```python
from build123d import *

# Parameters (mm, degrees)
SKETCH3_W                       = 80
SKETCH3_H                       = 80
SKETCH3_W_2                     = 60
SKETCH3_H_2                     = 60
BOSS_EXTRUDE2_DEPTH             = 1600
SKETCH7_W                       = 60
SKETCH7_H                       = 60
BOSS_EXTRUDE3_DEPTH             = 5
BOSS_EXTRUDE4_REACH             = 1610.361
SKETCH8_W                       = 105
SKETCH8_H                       = 5
BOSS_EXTRUDE4_DIRECTION_2_REACH = 1610.361
CUT_EXTRUDE1_DEPTH              = 5
CUT_EXTRUDE2_REACH              = 1612.59
FILLET1_R                       = 5
FILLET1_OF_MIRROR1_R            = 5
FILLET1_OF_MIRROR2_R            = 5


with BuildPart() as part:
    # Sketch3 → Boss-Extrude2 (new body)
    with BuildSketch(Plane(origin=(0, 0, 0), x_dir=(0, 0, -1), z_dir=(1, 0, 0))):
        with Locations((40, 40)):
            Rectangle(SKETCH3_W, SKETCH3_H)
        with Locations((40, 40)):
            Rectangle(SKETCH3_W_2, SKETCH3_H_2, mode=Mode.SUBTRACT)
    extrude(amount=BOSS_EXTRUDE2_DEPTH)

    # Sketch7 → Boss-Extrude3 (add)
    with BuildSketch(Plane(origin=(1495, 0, 0), x_dir=(0, 0, -1), z_dir=(1, 0, 0))):
        Polygon((-60, 85), (140, 85), (140, 5), (90, -35), (-10, -35), (-60, 5), align=None)
        with Locations((40, 40)):
            Rectangle(SKETCH7_W, SKETCH7_H, mode=Mode.SUBTRACT)
    boss_extrude3 = extrude(amount=BOSS_EXTRUDE3_DEPTH)

    # Boss-Extrude4: up to this face of the body (flat: up to its plane)
    boss_extrude4_end = Plane(part.part.faces().sort_by_distance((1497.5, 45, -140))[0])
    # Sketch8 → Boss-Extrude4 (add, up to the picked face)
    with BuildSketch(Plane(origin=(0, 0, -80), x_dir=(-1, 0, 0), z_dir=(0, 0, -1)), mode=Mode.PRIVATE) as boss_extrude4_sk1:
        with Locations((-1447.5, 82.5)):
            Rectangle(SKETCH8_W, SKETCH8_H)
    boss_extrude4_tool1 = split(extrude(boss_extrude4_sk1.sketch, amount=BOSS_EXTRUDE4_REACH, mode=Mode.PRIVATE), bisect_by=boss_extrude4_end, keep=Keep.BOTH, mode=Mode.PRIVATE)
    boss_extrude4 = boss_extrude4_tool1.solids().sort_by(Axis((1447.5, 82.5, -80), (0, 0, -1)))[0]
    add(boss_extrude4)

    # Boss-Extrude4 direction 2: up to this face of the body (flat: up to its plane)
    boss_extrude4_direction_2_end = Plane(part.part.faces().sort_by_distance((1497.5, 45, 60))[0])
    # Sketch8 → Boss-Extrude4 direction 2 (add, up to the picked face)
    with BuildSketch(Plane(origin=(0, 0, -80), x_dir=(-1, 0, 0), z_dir=(0, 0, -1)), mode=Mode.PRIVATE) as boss_extrude4_direction_2_sk1:
        with Locations((-1447.5, 82.5)):
            Rectangle(SKETCH8_W, SKETCH8_H)
    boss_extrude4_direction_2_tool1 = split(extrude(boss_extrude4_direction_2_sk1.sketch, amount=-BOSS_EXTRUDE4_DIRECTION_2_REACH, mode=Mode.PRIVATE), bisect_by=boss_extrude4_direction_2_end, keep=Keep.BOTH, mode=Mode.PRIVATE)
    boss_extrude4_direction_2 = boss_extrude4_direction_2_tool1.solids().sort_by(Axis((1447.5, 82.5, -80), (0, 0, 1)))[0]
    add(boss_extrude4_direction_2)

    # Sketch9 → Cut-Extrude1 (cut)
    with BuildSketch(Plane(origin=(0, 85, 0), x_dir=(1, 0, 0), z_dir=(0, 1, 0))):
        with BuildLine():
            Line((1395, 80), (1400.801257358, 71.298113962))
            ThreePointArc((1400.801257358, 71.298113962), (1403.927300662, 64.675212774), (1405, 57.430609057))
            Line((1405, 57.430609057), (1405, 22.569390943))
            ThreePointArc((1405, 22.569390943), (1403.927300662, 15.324787226), (1400.801257358, 8.701886038))
            Line((1400.801257358, 8.701886038), (1395, 0))
            Line((1395, 0), (1395, 80))
        make_face()
    cut_extrude1 = extrude(amount=-CUT_EXTRUDE1_DEPTH, mode=Mode.SUBTRACT)

    # Sketch10 → Cut-Extrude2 (cut, up to next)
    with BuildSketch(Plane(origin=(0, 85, 0), x_dir=(1, 0, 0), z_dir=(0, 1, 0)), mode=Mode.PRIVATE) as cut_extrude2_sk1:
        with BuildLine():
            Line((1412.5, 126.5), (1482.5, 126.5))
            ThreePointArc((1482.5, 126.5), (1489, 120), (1482.5, 113.5))
            Line((1482.5, 113.5), (1412.5, 113.5))
            ThreePointArc((1412.5, 113.5), (1406, 120), (1412.5, 126.5))
        make_face()
    cut_extrude2_tool1 = extrude(cut_extrude2_sk1.sketch, amount=-CUT_EXTRUDE2_REACH, mode=Mode.PRIVATE) & part.part
    # Sketch10 → Cut-Extrude2 (cut, up to next)
    with BuildSketch(Plane(origin=(0, 85, 0), x_dir=(1, 0, 0), z_dir=(0, 1, 0)), mode=Mode.PRIVATE) as cut_extrude2_sk2:
        with BuildLine():
            Line((1412.5, -33.5), (1482.5, -33.5))
            ThreePointArc((1482.5, -33.5), (1489, -40), (1482.5, -46.5))
            Line((1482.5, -46.5), (1412.5, -46.5))
            ThreePointArc((1412.5, -46.5), (1406, -40), (1412.5, -33.5))
        make_face()
    cut_extrude2_tool2 = extrude(cut_extrude2_sk2.sketch, amount=-CUT_EXTRUDE2_REACH, mode=Mode.PRIVATE) & part.part
    cut_extrude2_1 = cut_extrude2_tool1.solids().sort_by_distance((1447.5, 85, -120))[0]
    add(cut_extrude2_1, mode=Mode.SUBTRACT)
    cut_extrude2_2 = cut_extrude2_tool2.solids().sort_by_distance((1447.5, 85, 40))[0]
    add(cut_extrude2_2, mode=Mode.SUBTRACT)
    cut_extrude2 = cut_extrude2_1 + cut_extrude2_2  # Cut-Extrude2 as one shape, for the pattern or mirror that repeats it

    # Fillet1
    fillet1_edges = [part.edges().sort_by_distance(p)[0] for p in [
        (1500, 85, -40),
    ]]
    fillet(fillet1_edges, radius=FILLET1_R - 0.0001)  # a hair under: the kernel refuses the full size

    # Mirror1: Boss-Extrude3 across plane
    add(boss_extrude3.mirror(Plane(origin=(800, 0, 0), x_dir=(0, 0, 1), z_dir=(1, 0, 0))))

    # Fillet1 of Mirror1
    fillet1_of_mirror1_edges = [part.edges().sort_by_distance(p)[0] for p in [
        (100, 85, -40),
    ]]
    fillet(fillet1_of_mirror1_edges, radius=FILLET1_OF_MIRROR1_R - 0.0001)  # a hair under: the kernel refuses the full size

    # Mirror2: Boss-Extrude3, Boss-Extrude4, Boss-Extrude4 direction 2, Cut-Extrude1, Cut-Extrude2 across plane
    add(boss_extrude3.mirror(Plane(origin=(800, 0, 0), x_dir=(0, 0, 1), z_dir=(1, 0, 0))))
    add(boss_extrude4.mirror(Plane(origin=(800, 0, 0), x_dir=(0, 0, 1), z_dir=(1, 0, 0))))
    add(boss_extrude4_direction_2.mirror(Plane(origin=(800, 0, 0), x_dir=(0, 0, 1), z_dir=(1, 0, 0))))
    add(cut_extrude1.mirror(Plane(origin=(800, 0, 0), x_dir=(0, 0, 1), z_dir=(1, 0, 0))), mode=Mode.SUBTRACT)
    add(cut_extrude2.mirror(Plane(origin=(800, 0, 0), x_dir=(0, 0, 1), z_dir=(1, 0, 0))), mode=Mode.SUBTRACT)

    # Fillet1 of Mirror2
    fillet1_of_mirror2_edges = [part.edges().sort_by_distance(p)[0] for p in [
        (100, 85, -40),
    ]]
    fillet(fillet1_of_mirror2_edges, radius=FILLET1_OF_MIRROR2_R - 0.0001)  # a hair under: the kernel refuses the full size


solid = part.part
```
The listing builds one solid part. Answer for the finished solid, in the listing's coordinates (mm). A direction names the side the tool comes from. Coordinates: 2 decimals unless noted, no trailing zeros. Write each loop counter-clockwise with the first axis right and the second up, starting at its lowest first coordinate (ties: lowest second). Pieces come first, ordered by that corner, then holes. Notation, with made-up numbers: M 17.5,28 L 43.5,28 A18 cw 43.5,57 Z; hole C 35.5,2.5 d8. An arc over 180 degrees is marked long. Use a Markdown table: item, result. Add a question column.
1. Section C-C (y = -16.5) is taken. Give the vertices of the cut face in (x, z) (3 decimals).
2. Which of the six approach directions +Z, -Z, +X, -X, +Y, -Y give full straight-line access (tool end or side, diameter ignored) to faces 4 (the flat face through (1495, -2, -41)), 5 (the flat face through (1446, 80, -110)), 6 (the flat face through (49, 39, 0))?
3. For a pull along Z with two mould halves and no side action, classify faces 1 (the flat face through (789, 40, -10)), 2 (the flat face through (1600, 41, -4)), 3 (the flat face through (103, -15, -115)) as +Z half, -Z half, draft (parallel to the pull), parting line (faces both ways), or undercut.
4. Given P1, Ø18, axis at x = 698.5, y = 27, coming from the -Z side; P2, Ø12, axis at y = 45, z = -115.5, coming from the +X side; P3, Ø24, axis at x = 640, y = 35.5, coming from the +Z side, each flat-ended and moving along its own axis, determine where each tip first touches the part or whether it passes through.
5. Straight lines are drawn through the part: line 1 along X through (y, z) = (-25.5, -44.5); line 2 along Z through (x, y) = (442.5, 57); line 3 along Y through (x, z) = (936.5, -32). For each, find the intervals that lie inside material, in ascending order. Write a range as [from, to].
6. Section B-B (x = 423.5) is taken. Give the vertices of the cut face in (y, z).
7. Section A-A (y = 42.5) is taken. Give the vertices of the cut face in (x, z).
Data:
| question | item | result |
|---|---|---|
| 1 | outline | M 100,-113.125 L 105,-113.125 L 105,33.125 L 100,33.125 Z; M 1495,-113.125 L 1500,-113.125 L 1500,33.125 L 1495,33.125 Z |
| 2 | face 4 | -Y |
| 2 | face 5 | -Z, -Y |
| 2 | face 6 | +Z, -X, +Y, -Y |
| 3 | face 1 | undercut |
| 3 | face 2 | draft |
| 3 | face 3 | -Z half |
| 4 | P1 | stops at z = -80 |
| 4 | P2 | stops at x = 1500 |
| 4 | P3 | stops at z = 0 |
| 5 | line 1 | x = [100, 105], [1495, 1500] |
| 5 | line 2 | z = [-80, -70], [-10, 0] |
| 5 | line 3 | y = [0, 10], [70, 80] |
| 6 | outline | M 0,-80 L 80,-80 L 80,0 L 0,0 Z; hole M 10,-70 L 70,-70 L 70,-10 L 10,-10 Z |
| 7 | outline | M 0,-80 L 100,-80 L 100,-140 L 105,-140 L 105,-80 L 1495,-80 L 1495,-140 L 1500,-140 L 1500,-80 L 1600,-80 L 1600,-70 L 0,-70 Z; M 0,-10 L 1600,-10 L 1600,0 L 1500,0 L 1500,60 L 1495,60 L 1495,0 L 105,0 L 105,60 L 100,60 L 100,0 L 0,0 Z |
